Verification items for the finished model (mm, model axes). Face numbers are marked on the shaded views. Coordinates: 2 decimals unless noted, no trailing zeros. Order: outer loops, then holes, each group sorted by start corner. A loop starts at its lowest first (then second) coordinate and runs counter-clockwise, first axis right, second up. Notation, with made-up numbers: M 45.25,59 L 51.25,59 A17 cw 51.25,68 Z; hole C 28.25,45 d9. An arc over 180 degrees is marked long. Write item = value, one per line.
```python
from build123d import *

# Parameters (mm, degrees)
F0_R     = 4.75
F1_DEPTH = 2
F2_R     = 3.15
F3_DEPTH = 5.3
F4_R     = 2.3
F5_DEPTH = 7.301
F6_SIZE  = 0.3


with BuildPart() as f1:
    # F0 (on Top) → F1 (new body)
    with BuildSketch(Plane.XY):
        Circle(F0_R)
    extrude(amount=F1_DEPTH)

    # F2 (on face) → F3 (join)
    with BuildSketch(Plane.XY.offset(2)):
        Circle(F2_R)
    extrude(amount=F3_DEPTH)

    # F4 (on face) → F5 (cut, through all)
    with BuildSketch(Plane(origin=(0, 0, 0), x_dir=(1, 0, 0), z_dir=(0, 0, -1))):
        Circle(F4_R)
    extrude(amount=-F5_DEPTH, mode=Mode.SUBTRACT)

    # F6
    f6_edges = [f1.edges().sort_by_distance(p)[0] for p in [
        (-4.75, 0, 0),
        (-2.3, 0, 0),
        (-2.3, 0, 7.3),
        (-3.15, 0, 7.3),
        (-4.75, 0, 2),
    ]]
    chamfer(f6_edges, length=F6_SIZE)


solid = f1.part
```
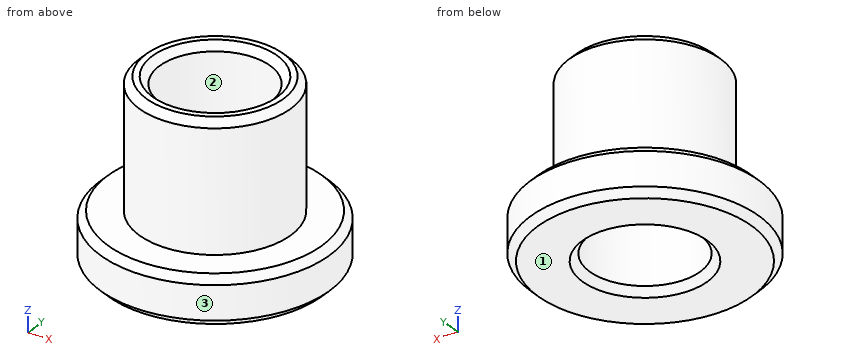
Item 1: Sectioned sample at A-A, the plane x = 0. Enter the section's corners in (y, z), then the cut area to 3 significant figures.
Report:
outline = M -4.75,0.3 L -4.45,0 L -2.6,0 L -2.3,0.3 L -2.3,7 L -2.6,7.3 L -2.85,7.3 L -3.15,7 L -3.15,2 L -4.45,2 L -4.75,1.7 Z; M 2.3,0.3 L 2.6,0 L 4.45,0 L 4.75,0.3 L 4.75,1.7 L 4.45,2 L 3.15,2 L 3.15,7 L 2.85,7.3 L 2.6,7.3 L 2.3,7 Z
area = 18.4 mm^2
Item 2: Sectioned sample at C-C, the plane z = 5. Enter the section's corners in (x, y), then the cut area to 3 significant figures.
Report:
outline = C 0,0 d6.3; hole C 0,0 d4.6
area = 14.6 mm^2
Item 3: Gauge pin test, flat ends, axial feed: pin 1 (4 mm diameter, centred on x = -4, z = 6.5, fed in from +Y); pin 2 (4 mm diameter, centred on y = 2, z = 3, fed in from -X); pin 3 (1 mm diameter, centred on x = 2, z = 3, fed in from -Y). Record the tip position at first contact, or that the pin passes through.
Report:
pin_1 = 2.43
pin_2 = -4.73
pin_3 = -2.77
Item 4: Scan lines: L1, parallel to Y at x = 0, z = 4.5; L2, parallel to Z at x = 2.5, y = 2; L3, parallel to Y at x = 1.5, z = 6. Record each from-to range of solid material in increasing order. Write a range as from..to.
Report:
L1 = -3.15..-2.3, 2.3..3.15
L2 = 0..2
L3 = -2.77..-1.74, 1.74..2.77
Item 5: Sectioned sample at D-D, the plane z = 1. Enter the section's corners in (x, y).
Report:
outline = C 0,0 d9.5; hole C 0,0 d4.6
Item 6: Release check for a two-part mould opening along X. For the marked faces 1, 2 and 3 record: pulls with the +X half, pulls with the -X half, needs draft (parallel to the pull), parting line crosses it, or undercut.
Report:
face_1 = needs draft
face_2 = undercut
face_3 = parting line crosses it
